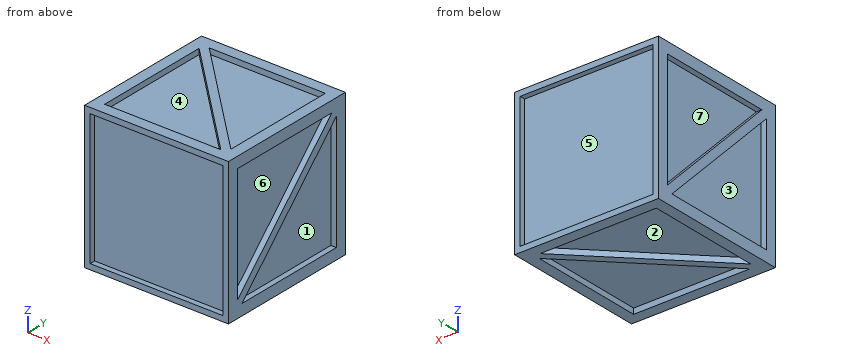
Autodesk Inventor part; units mm, degrees
ref_plane "YZ Plane" through (0, 0, 0) normal (1, 0, 0) x (0, 1, 0)
ref_plane "XZ Plane" through (0, 0, 0) normal (0, 1, 0) x (-1, 0, 0)
ref_plane "XY Plane" through (0, 0, 0) normal (0, 0, 1) x (1, 0, 0)
sketch "Sketch1" plane through (0, 0, 0) normal (0, 1, 0) x (-1, 0, 0)
  line L0 (158.5647, 157.6724) -> (-146.2353, 157.6724)
  line L1 (-146.2353, 157.6724) -> (-146.2353, -147.1276)
  line L2 (-146.2353, -147.1276) -> (158.5647, -147.1276)
  line L3 (158.5647, -147.1276) -> (158.5647, 157.6724)
  point P0 (0, 0)
  dimension "d0" = 304.8
  dimension "d1" = 304.8
extrude "Extrusion1" add sketch "Sketch1" along normal blind 304.8
sketch "Sketch2" plane through (146.2353, 0, 157.6724) normal (1, 0, 0) x (0, 0, -1)
  line L0 (-12.7, 317.5) -> (317.5, 317.5)
  line L1 (317.5, 317.5) -> (317.5, -12.7)
  line L2 (317.5, -12.7) -> (-12.7, -12.7)
  line L3 (-12.7, -12.7) -> (-12.7, 317.5)
  line L4 (0, 304.8) -> (304.8, 304.8)
  line L5 (0, 0) -> (0, 304.8)
  line L6 (12.7, 292.1) -> (292.1, 292.1)
  line L7 (292.1, 292.1) -> (292.1, 12.7)
  line L8 (292.1, 12.7) -> (12.7, 12.7)
  line L9 (12.7, 12.7) -> (12.7, 292.1)
  line L10 (25.4, 292.1) -> (292.1, 25.4)
  line L11 (279.4, 12.7) -> (12.7, 279.4)
  point P0 (157.6724, 0)
  dimension "d4" = 330.2
  dimension "d5" = 330.2
  dimension "d6" = 12.7
  dimension "d7" = 12.7
  dimension "d8" = 25.4
  dimension "d9" = 25.4
  dimension "d10" = 25.4
  dimension "d11" = 25.4
  dimension "d17" = 12.7
  dimension "d18" = 12.7
  dimension "d19" = 12.7
extrude "Extrusion2" add sketch "Sketch2" along normal blind 12.7 contours L0 L1 L2 L3 | L6 L10 L7 L8 L11 L9
ref_plane "Work Plane1" through (-6.1647, 0, -147.1276) normal (-1, 0, 0) x (0, 0, 1)
ref_plane "Work Plane2" through (-158.5647, 0, 5.2724) normal (0, 0, 1) x (1, 0, 0)
pattern_circular "Circular Pattern1" count 4 over 360 about axis through (-6.1647, 0, 5.2724) along (0, 1, 0) of "Extrusion2"
properties part number "cargoPrototype" material "Wood (Maple)"
Work out the finished part from the listing and answer in its coordinate system (mm). Face numbers are marked on the shaded views. A direction names the side the tool comes from. Give positions to 0.01 mm unless a question says otherwise; leave off trailing zeros. Write each loop counter-clockwise with the first axis right and the second up, starting at its lowest first coordinate (ties: lowest second). Pieces come first, ordered by that corner, then holes.
Q1. Given pin 1 (6 mm diameter, centred on x = -23.5, z = 77, fed in from -Y); pin 2 (1 mm diameter, centred on y = 221, z = 37.5, fed in from +X); pin 3 (3 mm diameter, centred on x = 20, y = 78, fed in from -Z), each flat-ended and moving along its own axis, determine where each tip first touches the part or whether it passes through.
Answer:
pin 1: stops at y = 0
pin 2: stops at x = 146.24
pin 3: stops at z = -147.13
Q2. The part is cut by section A-A on x = -139.5. Give the vertices of the cut face in (y, z).
Answer:
outline: (-12.7, -159.83) - (31.76, -159.83) - (31.76, -147.13) - (292.1, -147.13) - (292.1, -159.83) - (317.5, -159.83) - (317.5, -147.13) - (304.8, -147.13) - (304.8, 157.67) - (317.5, 157.67) - (317.5, 170.37) - (273.04, 170.37) - (273.04, 157.67) - (12.7, 157.67) - (12.7, 170.37) - (-12.7, 170.37) - (-12.7, 157.67) - (0, 157.67) - (0, -147.13) - (-12.7, -147.13) - close
Q3. Straight lines are drawn through the part: L1, parallel to Z at x = 17, y = 102.5; L2, parallel to X at y = 195, z = 22; L3, parallel to Y at x = 23, z = -64.5. For each, find the intervals that lie inside material, in ascending order.
Answer:
L1: z = -147.13 to 157.67
L2: x = -158.56 to 146.24
L3: y = 0 to 304.8
Q4. The part is cut by section C-C on x = -3. Give the vertices of the cut face in (y, z).
Answer:
outline: (-12.7, -159.83) - (12.7, -159.83) - (12.7, -147.13) - (142.86, -147.13) - (142.86, -159.83) - (168.26, -159.83) - (168.26, -147.13) - (292.1, -147.13) - (292.1, -159.83) - (317.5, -159.83) - (317.5, -147.13) - (304.8, -147.13) - (304.8, 157.67) - (317.5, 157.67) - (317.5, 170.37) - (292.1, 170.37) - (292.1, 157.67) - (161.94, 157.67) - (161.94, 170.37) - (136.54, 170.37) - (136.54, 157.67) - (12.7, 157.67) - (12.7, 170.37) - (-12.7, 170.37) - (-12.7, 157.67) - (0, 157.67) - (0, -147.13) - (-12.7, -147.13) - close
Q5. For a pull along X with two mould halves and no side action, classify the marked faces 5, 6 and 7 as released by +X, released by -X, zero draft, split by the parting line, or undercut.
Answer:
face 5: undercut
face 6: released by +X
face 7: released by -X
Q6. A tool of negligible diameter and unlimited length cuts with its end or side. For the marked faces 1, 2, 3 and 4, from which of +Z, -Z, +X, -X, +Y, -Y can it reach the whole face along a straight path? Write none if from no direction.
Answer:
face 1: +X
face 2: -Z
face 3: -X
face 4: +Z
Q7. The part is cut by section B-B on z = 30.5. Give the vertices of the cut face in (x, y), and give its area (3 significant figures).
Answer:
outline: (-171.26, -12.7) - (-158.56, -12.7) - (-158.56, 0) - (146.24, 0) - (146.24, -12.7) - (158.94, -12.7) - (158.94, 12.7) - (146.24, 12.7) - (146.24, 164.93) - (158.94, 164.93) - (158.94, 190.33) - (146.24, 190.33) - (146.24, 292.1) - (158.94, 292.1) - (158.94, 317.5) - (146.24, 317.5) - (146.24, 304.8) - (-158.56, 304.8) - (-158.56, 317.5) - (-171.26, 317.5) - (-171.26, 292.1) - (-158.56, 292.1) - (-158.56, 139.87) - (-171.26, 139.87) - (-171.26, 114.47) - (-158.56, 114.47) - (-158.56, 12.7) - (-171.26, 12.7) - close
area: 94,800 mm2
